Study the drawing (mm; zero at the part's minimum x, y, z) and answer. Coordinates: 2 decimals unless noted, no trailing zeros. Loops run counter-clockwise (first coordinate to the right, second up) from the corner with the lowest first, then second, coordinate; pieces in that order, holes last. Notation, with made-up numbers: M 0,23.25 L 18,23.25 A28 cw 18,49.25 Z; hole C 79,74.5 d2. An arc over 180 degrees is marked long. Use one line per item in the form item = value. Start each with the question number.
1. Flat-ended cylindrical pins translate along their axes: pin 1 (0.6 mm diameter, centred on x = 1, y = 1, fed in from +Z); pin 2 (0.6 mm diameter, centred on x = 1, y = 1.5, fed in from -Z); pin 3 (1.5 mm diameter, centred on y = 2, z = 214, fed in from -X). Find the tip coordinate at first contact, or state that the pin passes through.
2. Find the intervals of material crossed by probe 1 along Z at (x, y) = (8, 0.4), in increasing order. Write a range as [from, to].
3. The part is cut by section A-A (y = 0.5). Give the vertices of the cut face in (x, z).
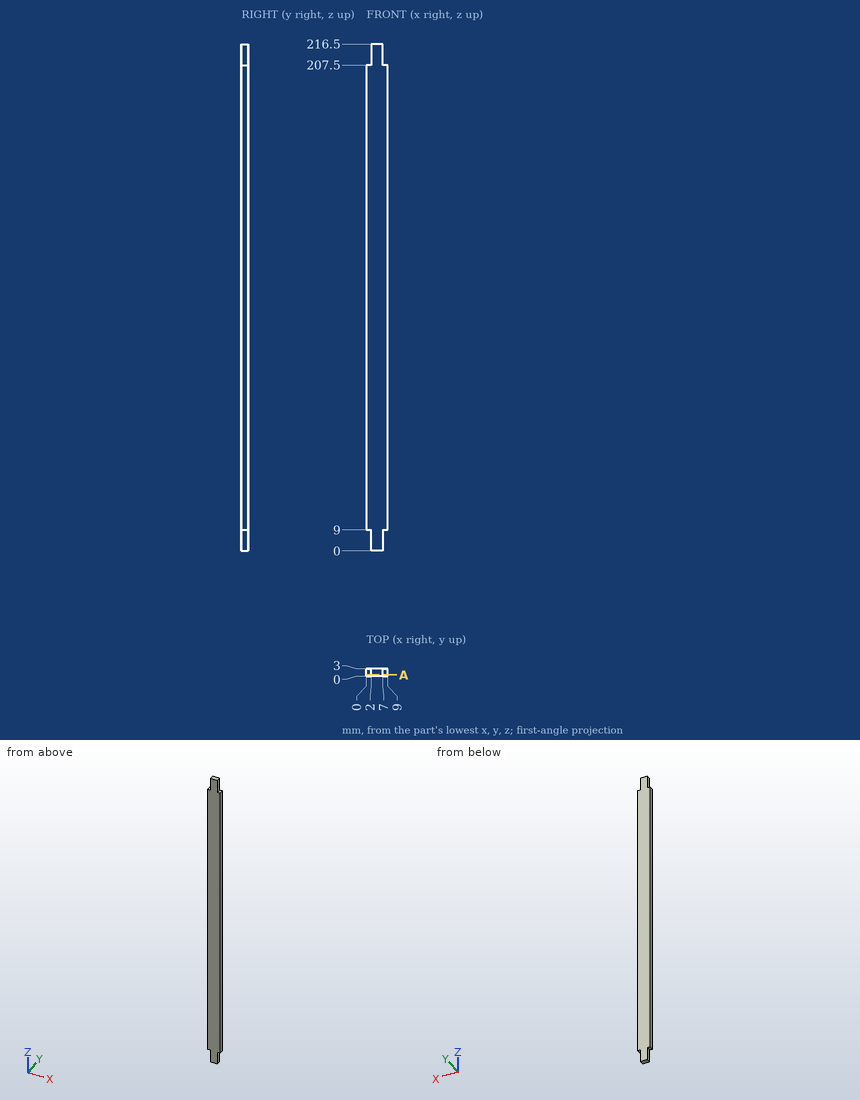
Computed values:
q1.pin_1 = 207.5
q1.pin_2 = 9
q1.pin_3 = 2
q2.probe_1 = [9, 207.5]
q3.outline = M 0,9 L 2,9 L 2,0 L 7,0 L 7,9 L 9,9 L 9,207.5 L 7,207.5 L 7,216.5 L 2,216.5 L 2,207.5 L 0,207.5 Z
